Could you check a few things on this model? Use its own coordinates, in mm. A direction names the side the tool comes from. Give positions to 0.01 mm unless a question says otherwise; leave off trailing zeros. Write each loop counter-clockwise with the first axis right and the second up, starting at its lowest first coordinate (ties: lowest second). Pieces come first, ordered by that corner, then holes. Notation, with made-up numbers: (84, 45.25) - (119, 45.25) arc R23 ccw to (119, 74.25) - close; hole circle Ø3 at (61.25, 82). An arc over 180 degrees is marked (long way). Use one line per item in the form item = value.
```python
from build123d import *

# Parameters (mm, degrees)
SKETCH_W        = 30
SKETCH_H        = 20
PAD_DEPTH       = 5
SKETCH001_R     = 2.65
POCKET_DEPTH    = 5
SKETCH002_W     = 15
SKETCH002_H     = 20
PAD001_DEPTH    = 20
SKETCH003_R     = 9
POCKET001_DEPTH = 15
FILLET_R        = 9.99


with BuildPart() as part:
    # Sketch → Pad (new body)
    with BuildSketch(Plane.XY):
        Rectangle(SKETCH_W, SKETCH_H)
    extrude(amount=PAD_DEPTH)

    # Sketch001 (on Face6 of Pad) → Pocket (cut)
    with BuildSketch(Plane.XY.offset(5)):
        with Locations((-7.5, 0)):
            Circle(SKETCH001_R)
    extrude(amount=-POCKET_DEPTH, mode=Mode.SUBTRACT)

    # Sketch002 (on Face5 of Pocket) → Pad001 (join)
    with BuildSketch(Plane.XY.offset(5)):
        with Locations((7.5, 0)):
            Rectangle(SKETCH002_W, SKETCH002_H)
    extrude(amount=PAD001_DEPTH)

    # Sketch003 (on Face11 of Pad001) → Pocket001 (cut)
    with BuildSketch(Plane.YZ.offset(15)):
        with Locations((0, 15)):
            Circle(SKETCH003_R)
    extrude(amount=-POCKET001_DEPTH, mode=Mode.SUBTRACT)

    # Fillet
    fillet_edges = [part.edges().sort_by_distance(p)[0] for p in [
        (7.5, -10, 25),
        (7.5, 10, 25),
    ]]
    fillet(fillet_edges, radius=FILLET_R)


solid = part.part
```
1. If we mould it in two halves opening along Y, with no side actions, what happens to faces 3 (the face through (-15, 0, 2)), 4 (the face through (3, -10, 6)), 5 (the face through (7.605, -1.172, 23.923))? For each: pulls with the +Y half, pulls with the -Y half, needs draft (parallel to the pull), parting line crosses it, or undercut.
Response values:
face_3 = needs draft
face_4 = pulls with the -Y half
face_5 = undercut
2. If I drill on line 1 (Y direction, x = -7.5, z = 1.4); line 2 (Z direction, x = 6.75, y = 0); line 3 (Z direction, x = -9, y = -6.75), over which ranges is the centre line in solid material (lowest first)? Write a range as from..to.
Response values:
line_1 = -10..-2.65, 2.65..10
line_2 = 0..6, 24..25
line_3 = 0..5
3. For pin 1 (10 mm diameter, centred on x = -3, y = -0.5, fed in from +Z); pin 2 (10 mm diameter, centred on y = -4, z = 18.5, fed in from -X); pin 3 (8.5 mm diameter, centred on x = -7.5, y = 0, fed in from +Z); pin 4 (1 mm diameter, centred on x = 7.5, y = 4.5, fed in from +Z), each with a flat end and sliding along its axis, tell me the tip position at first contact or that it passes through.
Response values:
pin_1 = 25
pin_2 = 0
pin_3 = 5
pin_4 = 24.17
4. Imagine slicing it at C-C, the plane x = -7.5. List the corners of the cut face in (y, z) for me, and give its area (3 significant figures).
Response values:
outline = (-10, 0) - (-2.65, 0) - (-2.65, 5) - (-10, 5) - close; (2.65, 0) - (10, 0) - (10, 5) - (2.65, 5) - close
area = 73.5 mm²
5. Imagine slicing it at B-B, the plane z = 4.5. List the corners of the cut face in (x, y) for me, and give its area (3 significant figures).
Response values:
outline = (-15, -10) - (15, -10) - (15, 10) - (-15, 10) - close; hole circle Ø5.3 at (-7.5, 0)
area = 578 mm²
6. Which directions (+Z, -Z, +X, -X, +Y, -Y) give clear straight access to the entire face, cutting with the end or side of a thin tool? Please do faces 1 (the face through (7.6, 7, 22.15)), 2 (the face through (-9.3, 2.4, 5)).
Response values:
face_1 = +Z, +X, -X, +Y
face_2 = +Z, -X, +Y, -Y
7. Imagine slicing it at D-D, the plane y = 1.5. List the corners of the cut face in (x, z) for me, and give its area (3 significant figures).
Response values:
outline = (-15, 0) - (-9.68, 0) - (-9.68, 5) - (-15, 5) - close; (-5.32, 0) - (15, 0) - (15, 6.13) - (0, 6.13) - (0, 5) - (-5.32, 5) - close; (0, 23.87) - (15, 23.87) - (15, 24.89) - (0, 24.89) - close
area = 160 mm²
